```python
from build123d import *

# Parameters (mm, degrees)
SKETCH_1_R                           = 3.75
EXTRUDE_1_DEPTH                      = 7.5
EXTRUDE_2_DEPTH                      = 2
EXTRUDE_2_DEPTH_BACK                 = 2
CUT_EXTRUDE_1_DEPTH                  = 2
CUT_EXTRUDE_1_DEPTH_BACK             = 2
CUT_EXTRUDE_2_REACH                  = 11.186
CUT_EXTRUDE_2_END_RADIUS             = 3.75
CUT_EXTRUDE_2_DIRECTION_2_REACH      = 11.186
CUT_EXTRUDE_2_DIRECTION_2_END_RADIUS = 3.75
FILLET_1_R                           = 0.1
SKETCH_5_R                           = 0.75
CUT_EXTRUDE_3_DEPTH                  = 6
CHAMFER_1_SIZE                       = 0.2


with BuildPart() as part:
    # 草图1 → 凸台-拉伸1 (new body)
    with BuildSketch(Plane(origin=(0, 0, 0), x_dir=(1, 0, 0), z_dir=(0, 1, 0))):
        with Locations(Location((0, 0, 0), (0, 0, 270))):
            Circle(SKETCH_1_R)
    extrude(amount=-EXTRUDE_1_DEPTH)

    # 草图2 → 凸台-拉伸2 (add, two sides: drawn at the far end of the back side and taken through both)
    with BuildSketch(Plane.XY.offset(-EXTRUDE_2_DEPTH_BACK)):
        with BuildLine():
            Line((-1.95, 2.5), (1.95, 2.5))
            Line((1.95, 2.5), (1.95, 1.555590279))
            ThreePointArc((1.95, 1.555590279), (1.780042303, 1.088161527), (1.5, 0.677124344))
            Line((1.5, 0.677124344), (1.5, 0))
            Line((1.5, 0), (-1.5, 0))
            Line((-1.5, 0), (-1.5, 0.677124344))
            ThreePointArc((-1.5, 0.677124344), (-1.780042303, 1.088161527), (-1.95, 1.555590279))
            Line((-1.95, 1.555590279), (-1.95, 2.5))
        make_face()
    extrude(amount=EXTRUDE_2_DEPTH + EXTRUDE_2_DEPTH_BACK)

    # 草图3 → 切除-拉伸1 (cut, two sides: drawn at the far end of the back side and taken through both)
    with BuildSketch(Plane(origin=(0, 0, 0), x_dir=(0, 0, -1), z_dir=(1, 0, 0)).offset(-CUT_EXTRUDE_1_DEPTH_BACK)):
        with BuildLine():
            Line((1.95, 2.5), (1.95, 1.555590279))
            ThreePointArc((1.95, 1.555590279), (1.780042303, 1.088161527), (1.5, 0.677124344))
            Line((1.5, 0.677124344), (1.5, 0))
            Line((1.5, 0), (2, 0))
            Line((2, 0), (2, 2.5))
            Line((2, 2.5), (1.95, 2.5))
        make_face()
        with BuildLine():
            Line((-2, 0), (-1.5, 0))
            Line((-1.5, 0), (-1.5, 0.677124344))
            ThreePointArc((-1.5, 0.677124344), (-1.780042303, 1.088161527), (-1.95, 1.555590279))
            Line((-1.95, 1.555590279), (-1.95, 2.5))
            Line((-1.95, 2.5), (-2, 2.5))
            Line((-2, 2.5), (-2, 0))
        make_face()
    extrude(amount=CUT_EXTRUDE_1_DEPTH + CUT_EXTRUDE_1_DEPTH_BACK, mode=Mode.SUBTRACT)

    # 切除-拉伸2: up to this cylinder (the profile starts inside it)
    cut_extrude_2_end = Plane(origin=(0, -5.585293, 0), z_dir=(0, 1, 0)) * Cylinder(CUT_EXTRUDE_2_END_RADIUS, 30.872, mode=Mode.PRIVATE)
    # 草图4 → 切除-拉伸2 (cut, up to the surface)
    with BuildSketch(Plane.XY, mode=Mode.PRIVATE) as cut_extrude_2_sk1:
        with BuildLine():
            Line((-1.5, -7.5), (1.5, -7.5))
            Line((1.5, -7.5), (1.5, -6.822875656))
            ThreePointArc((1.5, -6.822875656), (0, -3.5), (-1.5, -6.822875656))
            Line((-1.5, -6.822875656), (-1.5, -7.5))
        make_face()
    cut_extrude_2_tool1 = extrude(cut_extrude_2_sk1.sketch, amount=-CUT_EXTRUDE_2_REACH, mode=Mode.PRIVATE) & cut_extrude_2_end
    add(cut_extrude_2_tool1.solids().sort_by_distance((0, -5.585293, 0))[0], mode=Mode.SUBTRACT)

    # 切除-拉伸2 direction 2: up to this cylinder (the profile starts inside it)
    cut_extrude_2_direction_2_end = Plane(origin=(0, -5.585293, 0), z_dir=(0, 1, 0)) * Cylinder(CUT_EXTRUDE_2_DIRECTION_2_END_RADIUS, 30.872, mode=Mode.PRIVATE)
    # 草图4 → 切除-拉伸2 direction 2 (cut, up to the surface)
    with BuildSketch(Plane.XY, mode=Mode.PRIVATE) as cut_extrude_2_direction_2_sk1:
        with BuildLine():
            Line((-1.5, -7.5), (1.5, -7.5))
            Line((1.5, -7.5), (1.5, -6.822875656))
            ThreePointArc((1.5, -6.822875656), (0, -3.5), (-1.5, -6.822875656))
            Line((-1.5, -6.822875656), (-1.5, -7.5))
        make_face()
    cut_extrude_2_direction_2_tool1 = extrude(cut_extrude_2_direction_2_sk1.sketch, amount=CUT_EXTRUDE_2_DIRECTION_2_REACH, mode=Mode.PRIVATE) & cut_extrude_2_direction_2_end
    add(cut_extrude_2_direction_2_tool1.solids().sort_by_distance((0, -5.585293, 0))[0], mode=Mode.SUBTRACT)

    # 圆角1
    fillet_1_edges = [part.edges().sort_by_distance(p)[0] for p in [
        (0, 2.5, 1.95),
        (1.95, 2.5, 0),
        (-1.95, 2.5, 0),
        (0, 2.5, -1.95),
    ]]
    fillet(fillet_1_edges, radius=FILLET_1_R)

    # 草图5 → 切除-拉伸3 (cut)
    with BuildSketch(Plane.XZ.offset(7.5)):
        with Locations(Location((0, 0, 0), (0, 0, 270))):
            Circle(SKETCH_5_R)
    extrude(amount=-CUT_EXTRUDE_3_DEPTH, mode=Mode.SUBTRACT)

    # 倒角1
    chamfer_1_edges = [part.edges().sort_by_distance(p)[0] for p in [
        (0, 0, -3.75),
        (3.75, -7.5, 0),
        (-3.75, -7.5, 0),
    ]]
    chamfer(chamfer_1_edges, length=CHAMFER_1_SIZE)


solid = part.part
```
Verification items for the finished model (mm, model axes). A direction names the side the tool comes from. Coordinates: 2 decimals unless noted, no trailing zeros. Order: outer loops, then holes, each group sorted by start corner. A loop starts at its lowest first (then second) coordinate and runs counter-clockwise, first axis right, second up. Notation, with made-up numbers: (34.25, -40) -> (50.25, -40) arc R13 cw to (50.25, -19) -> close; hole circle Ø7 at (82, -7). An arc over 180 degrees is marked (long way). Put each result on its own line as item: value. Start each with the question number.
1) Cross-section at A-A (z = 0). Enter the section's corners in (x, y).
2) Release check for a two-part mould opening along Z. For faces 4 (the flat face through (0, -1.5, 0)), 5 (the cylindrical face through (0.165, -2.911, -3.746)), 6 (the flat face through (-1.95, 2, 0)) record: pulls with the +Z half, pulls with the -Z half, needs draft (parallel to the pull), parting line crosses it, or undercut.
3) Cross-section at C-C (y = -4.5). Enter the section's corners in (x, z), plus the area to 3 significant figures.
4) Go/stop test with flat-tipped pins: pin 1 (1.7 mm diameter, centred on x = 0, z = 0, fed in from -Y); pin 2 (0.7 mm diameter, centred on y = 2, z = 0, fed in from -X); pin 3 (0.7 mm diameter, centred on y = 0.5, z = -0.5, fed in from -X). Record where each tip stops, or that it passes through.
5) Tool access check on faces 1 (the cylindrical face through (-0.03, 1.09, -1.78)), 2 (the cylindrical face through (1.78, 1.09, -0.03)), 3 (the flat face through (0, 2, 1.95)). Record the directions out of +Z, -Z, +X, -X, +Y, -Y that give a thin tool (end or side, any length) a straight path to the whole face; none if there is none.
6) Cross-section at B-B (y = -3). Enter the section's corners in (x, z), plus the area to 3 significant figures.
7) Material ranges on L1, parallel to X at y = -2, z = 0; L2, parallel to X at y = -5.5, z = 1.5; L3, parallel to Y at x = 2.5, z = 1.5, recorded low to high.
8) Cross-section at D-D (y = 0.25). Enter the section's corners in (x, z).
Geometry check:
1. outline: (-3.75, -7.3) -> (-3.55, -7.5) -> (-1.5, -7.5) -> (-1.5, -6.82) arc R2 cw to (-0.75, -3.65) -> (-0.75, -1.5) -> (0.75, -1.5) -> (0.75, -3.65) arc R2 cw to (1.5, -6.82) -> (1.5, -7.5) -> (3.55, -7.5) -> (3.75, -7.3) -> (3.75, -0.2) -> (3.55, 0) -> (1.5, 0) -> (1.5, 0.68) arc R2 ccw to (1.95, 1.56) -> (1.95, 2.4) arc R0.1 ccw to (1.85, 2.5) -> (-1.85, 2.5) arc R0.1 ccw to (-1.95, 2.4) -> (-1.95, 1.56) arc R2 ccw to (-1.5, 0.68) -> (-1.5, 0) -> (-3.55, 0) -> (-3.75, -0.2) -> close
2. face 4: undercut
2. face 5: parting line crosses it
2. face 6: needs draft
3. outline: (-1.73, -3.33) -> (-1.73, 3.33) arc R3.75 ccw to start; (1.73, -3.33) arc R3.75 ccw to (1.73, 3.33) -> close
3. area: 19.2 mm^2
4. pin 1: stops at y = -3.69
4. pin 2: stops at x = -1.95
4. pin 3: stops at x = -1.64
5. face 1: -Z, +X, -X
5. face 2: +Z, -Z, +X
5. face 3: +Z, +X, -X, +Y
6. outline: circle Ø7.5 at (0, 0); hole circle Ø1.5 at (0, 0)
6. area: 42.4 mm^2
7. L1: x = -3.75 to -0.75, 0.75 to 3.75
7. L2: x = -3.44 to -2, 2 to 3.44
7. L3: y = -7.5 to 0
8. outline: (-1.5, -1.5) -> (1.5, -1.5) -> (1.5, 1.5) -> (-1.5, 1.5) -> close
